Could you check a few things on this model? Use its own coordinates, in mm. Face numbers are marked on the shaded views. Round coordinates to 2 decimals unless told otherwise and drop trailing zeros. Order: outer loops, then holes, each group sorted by start corner. A loop starts at its lowest first (then second) coordinate and runs counter-clockwise, first axis right, second up. Notation, with made-up numbers: (-19, -3) - (16, -3) arc R17 cw to (16, 8) - close; hole circle Ø1 at (70.25, -9.75). An arc over 180 degrees is marked (long way). Return JSON: item names as keys, results as strings. Group by question number.
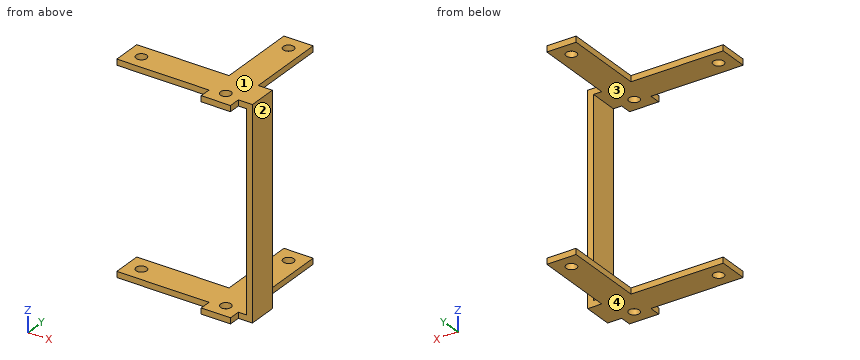
from build123d import *

# Parameters (mm, degrees)
SKETCH1_R           = 4.5
BOSS_EXTRUDE1_DEPTH = 5
SKETCH2_W           = 5
SKETCH2_H           = 25
BOSS_EXTRUDE2_DEPTH = 83.5


with BuildPart() as part:
    # Sketch1 → Boss-Extrude1 (new body)
    with BuildSketch(Plane.XY):
        Polygon((0, 0), (-78.75, 0), (-78.75, -25), (0, -25), (0, -34.8), (25, -34.8), (25, -25), (37, -25), (37, 0), (25, 0), (25, 68.7), (0, 68.7), align=None)
        with Locations((-66.25, -12.5)):
            Circle(SKETCH1_R, mode=Mode.SUBTRACT)
        with Locations((12.5, -22.3)):
            Circle(SKETCH1_R, mode=Mode.SUBTRACT)
        with Locations((12.5, 56.2)):
            Circle(SKETCH1_R, mode=Mode.SUBTRACT)
    extrude(amount=BOSS_EXTRUDE1_DEPTH)

    # Sketch2 → Boss-Extrude2 (add)
    with BuildSketch(Plane(origin=(0, 0, 0), x_dir=(-1, 0, 0), z_dir=(0, 0, -1))):
        with Locations((-34.5, -12.5)):
            Rectangle(SKETCH2_W, SKETCH2_H)
    extrude(amount=BOSS_EXTRUDE2_DEPTH)

    # Mirror5: part across plane


with BuildPart() as part_1:
    add(part.part)
    add(part.part.mirror(Plane(origin=(0, 0, -83.5), x_dir=(1, 0, 0), z_dir=(0, 0, -1))))


solid = part_1.part
1) I want a section at C-C, the plane y = -22.3. List the corners of the cut face in (x, z) for me.
2) Will these pins go through, and if not, where does the flat tip stop? pin 1 (10.5 mm diameter, centred on x = 12.5, y = 56.2, fed in from -Z); pin 2 (13 mm diameter, centred on x = 33.5, z = -51.5, fed in from -Y); pin 3 (12.5 mm diameter, centred on y = -9.5, z = -76, fed in from -X); pin 4 (1.5 mm diameter, centred on x = -42.5, z = -170, fed in from +Y).
3) If I drill on line 1 along Y through (x, z) = (12, -169); line 2 along Z through (x, y) = (-33.5, -13); line 3 along X through (y, z) = (-12, 3), over which ranges is the centre line in solid material (lowest first)? Write a range as from..to.
4) We'd pull the mould along Z, two halves only. Please class the marked faces 1, 2, 3 and 4: +Z half, -Z half, draft (parallel to the pull), parting line (faces both ways), or undercut.
5) I want a section at A-A, the plane y = 46.5. List the corners of the cut face in (x, z) for me, plus the area to 3 significant figures.
6) I want a section at D-D, the plane x = -66.25. List the corners of the cut face in (y, z) for me.
7) I want a section at B-B, the plane x = -17.5. List the corners of the cut face in (y, z) for me, plus the area to 3 significant figures.
Outcome:
{
 "1": {"outline": "(-78.75, -172) - (8, -172) - (8, -167) - (-78.75, -167) - close; (-78.75, 0) - (8, 0) - (8, 5) - (-78.75, 5) - close; (17, -172) - (37, -172) - (37, 5) - (17, 5) - (17, 0) - (32, 0) - (32, -167) - (17, -167) - close"},
 "2": {"pin 1": "z = -172", "pin 2": "y = -25", "pin 3": "x = 32", "pin 4": "y = 0"},
 "3": {"line 1": "-34.8..-26.77, -17.83..51.73, 60.67..68.7", "line 2": "-172..-167, 0..5", "line 3": "-78.75..-70.72, -61.78..37"},
 "4": {"face 1": "+Z half", "face 2": "draft", "face 3": "undercut", "face 4": "-Z half"},
 "5": {"outline": "(0, -172) - (25, -172) - (25, -167) - (0, -167) - close; (0, 0) - (25, 0) - (25, 5) - (0, 5) - close", "area": "250 mm^2"},
 "6": {"outline": "(-25, -172) - (-17, -172) - (-17, -167) - (-25, -167) - close; (-25, 0) - (-17, 0) - (-17, 5) - (-25, 5) - close; (-8, -172) - (0, -172) - (0, -167) - (-8, -167) - close; (-8, 0) - (0, 0) - (0, 5) - (-8, 5) - close"},
 "7": {"outline": "(-25, -172) - (0, -172) - (0, -167) - (-25, -167) - close; (-25, 0) - (0, 0) - (0, 5) - (-25, 5) - close", "area": "250 mm^2"}
}
